Here's how the part is built. I have some questions about the finished solid (model axes, mm). A direction names the side the tool comes from. Round coordinates to 2 decimals unless told otherwise and drop trailing zeros. Order: outer loops, then holes, each group sorted by start corner. A loop starts at its lowest first (then second) coordinate and runs counter-clockwise, first axis right, second up. Notation, with made-up numbers: (42, 63.5) -> (60, 63.5) arc R15 ccw to (60, 85.5) -> close; hole circle Ø2 at (8.5, 20.25). An arc over 180 degrees is marked (long way). Use a Markdown table: item, result. Add a question column.
(1) I want a section at B-B, the plane z = 15. Please give me the cut outline in (x, y), then the cut area to 3 significant figures.
(2) I want a section at C-C, the plane x = 57.5. Please give me the cut outline in (y, z), then the cut area to 3 significant figures.
(3) I want a section at D-D, the plane y = -17. Please give me the cut outline in (x, z).
(4) I'm going to push flat-ended pins straight in: P1, Ø2, axis at x = 85.5, y = 9.5, coming from the -Z side; P2, Ø11.5, axis at x = -31.89, y = 0, coming from the -Z side; P3, Ø1, axis at y = -3.5, z = -4, coming from the -X side. Where does each tip first touch, or does it pass through?
(5) I want a section at A-A, the plane y = 0. Please give me the cut outline in (x, z), then the cut area to 3 significant figures.
(6) On a 3-axis mill with a long thin cutter (end or side, diameter ignored), from which of +Z, -Z, +X, -X, +Y, -Y can I reach the whole of each face in a straight line? I mean faces 4 (the face through (-1, 0, 30)), 5 (the face through (60, -5, 18)), 6 (the face through (107, 0, 20)), 7 (the face through (45, 0, 20)). Say none if no direction works.
(7) If I drill on probe 1 along Y at (x, z) = (44, 15); probe 2 along X at (y, z) = (-13, 8); probe 3 along X at (y, z) = (-11, -21.5), over which ranges is the centre line in solid material (lowest first)?
(8) Thinking about a two-plate mould opening in X: for faces 1 (the face through (78.73, -0.28, -30.79)), 2 (the face through (34, -20, 2)), 3 (the face through (-60, 0, 15)), which applies, pulls with the +X half, pulls with the -X half, needs draft (parallel to the pull), parting line crosses it, or undercut?
from build123d import *

# Parameters (mm, degrees)
BOSS_EXTRU_1_DEPTH      = 30
ESQUISSE3_R             = 5
ENL_V_MAT_EXTRU_1_DEPTH = 40
ESQUISSE4_R             = 5
ENL_V_MAT_EXTRU_2_DEPTH = 30
EXTRU_MINCE1_DEPTH      = 20


with BuildPart() as part:
    # Esquisse1 → Boss.-Extru.1 (new body)
    with BuildSketch(Plane.XY):
        with BuildLine():
            Line((-50, -20), (60, -20))
            Line((60, -20), (60, 20))
            Line((60, 20), (-50, 20))
            ThreePointArc((-50, 20), (-57.071067812, 17.071067812), (-60, 10))
            Line((-60, 10), (-60, -10))
            ThreePointArc((-60, -10), (-57.071067812, -17.071067812), (-50, -20))
        make_face()
    extrude(amount=BOSS_EXTRU_1_DEPTH)

    # Esquisse3 → Enlèv. mat.-Extru.1 (cut)
    with BuildSketch(Plane(origin=(0, 0, 0), x_dir=(-1, 0, 0), z_dir=(0, 0, -1))):
        with Locations((31.886780036, 0)):
            Circle(ESQUISSE3_R)
    extrude(amount=-ENL_V_MAT_EXTRU_1_DEPTH, mode=Mode.SUBTRACT)

    # Esquisse4 → Enlèv. mat.-Extru.2 (cut)
    with BuildSketch(Plane(origin=(60, 0, 0), x_dir=(0, 0, -1), z_dir=(1, 0, 0))):
        with Locations((-15, 0)):
            Circle(ESQUISSE4_R)
    extrude(amount=-ENL_V_MAT_EXTRU_2_DEPTH, mode=Mode.SUBTRACT)

    # Esquisse11 → Extru.-Mince1 (add, symmetric)
    with BuildSketch(Plane(origin=(0, 0, 0), x_dir=(-1, 0, 0), z_dir=(0, -1, 0))):
        with BuildLine():
            ThreePointArc((-60, 0), (-77.250281864, 17.250281864), (-94.500563727, 0))
            Line((-94.500563727, 0), (-94.500563727, -30))
            Line((-94.500563727, -30), (-120.200563727, -30))
            Line((-120.200563727, -30), (-120.200563727, 0))
            ThreePointArc((-120.200563727, 0), (-79.40232614, 40.798237588), (-38.604088552, 0))
            Line((-38.604088552, 0), (-48.604088552, 0))
            ThreePointArc((-48.604088552, 0), (-79.40232614, 30.798237588), (-110.200563727, 0))
            Line((-110.200563727, 0), (-110.200563727, -20))
            Line((-110.200563727, -20), (-104.500563727, -20))
            Line((-104.500563727, -20), (-104.500563727, 0))
            ThreePointArc((-104.500563727, 0), (-77.250281864, 27.250281864), (-50, 0))
            Line((-50, 0), (-60, 0))
        make_face()
    extrude(amount=EXTRU_MINCE1_DEPTH, both=True)


solid = part.part
Taken from the geometry:
| question | item | result |
|---|---|---|
| 1 | outline | (-60, -10) arc R10 ccw to (-50, -20) -> (60, -20) -> (60, -5) -> (30, -5) -> (30, 5) -> (60, 5) -> (60, 20) -> (-50, 20) arc R10 ccw to (-60, 10) -> close; (94.5, -20) -> (104.5, -20) -> (104.5, 20) -> (94.5, 20) -> close; (110.2, -20) -> (120.2, -20) -> (120.2, 20) -> (110.2, 20) -> close; hole circle Ø10 at (-31.89, 0) |
| 1 | area | 5,180 mm2 |
| 2 | outline | (-20, -34.42) -> (20, -34.42) -> (20, -21.65) -> (-20, -21.65) -> close; (-20, -18.78) -> (20, -18.78) -> (20, 30) -> (-20, 30) -> close; hole circle Ø10 at (0, 15) |
| 2 | area | 2,380 mm2 |
| 3 | outline | (-57.14, 0) -> (38.6, 0) arc R40.8 ccw to (120.2, 0) -> (120.2, 30) -> (94.5, 30) -> (94.5, 0) arc R17.25 cw to (60, 0) -> (60, 30) -> (-57.14, 30) -> close; hole (48.6, 0) arc R30.8 ccw to (110.2, 0) -> (110.2, 20) -> (104.5, 20) -> (104.5, 0) arc R27.25 cw to (50, 0) -> close |
| 4 | P1 | stops at z = -40.48 |
| 4 | P2 | stops at z = 0 |
| 4 | P3 | stops at x = 38.75 |
| 5 | outline | (-60, 0) -> (-36.89, 0) -> (-36.89, 30) -> (-60, 30) -> close; (-26.89, 0) -> (38.6, 0) arc R40.8 ccw to (120.2, 0) -> (120.2, 30) -> (94.5, 30) -> (94.5, 0) arc R17.25 cw to (60, 0) -> (60, 10) -> (30, 10) -> (30, 20) -> (60, 20) -> (60, 30) -> (-26.89, 30) -> close; hole (48.6, 0) arc R30.8 ccw to (110.2, 0) -> (110.2, 20) -> (104.5, 20) -> (104.5, 0) arc R27.25 cw to (50, 0) -> close |
| 5 | area | 5,480 mm2 |
| 6 | face 4 | +Z, +X, -X, +Y, -Y |
| 6 | face 5 | +Z, +Y, -Y |
| 6 | face 6 | +Y, -Y |
| 6 | face 7 | none |
| 7 | probe 1 | y = -20 to -5, 5 to 20 |
| 7 | probe 2 | x = -59.54 to 60, 94.5 to 104.5, 110.2 to 120.2 |
| 7 | probe 3 | x = 44.73 to 57.35, 60.51 to 93.99, 101.45 to 114.08 |
| 8 | face 1 | undercut |
| 8 | face 2 | needs draft |
| 8 | face 3 | pulls with the -X half |
